Autodesk Inventor part; units mm, degrees
ref_plane "YZ Plane" through (0, 0, 0) normal (1, 0, 0) x (0, 1, 0)
ref_plane "XZ Plane" through (0, 0, 0) normal (0, 1, 0) x (-1, 0, 0)
ref_plane "XY Plane" through (0, 0, 0) normal (0, 0, 1) x (1, 0, 0)
sketch "Sketch1" plane through (0, 0, 0) normal (0, 0, 1) x (1, 0, 0)
  line L0 (-160, -10) -> (160, -10)
  line L1 (160, -10) -> (160, 10) construction
  line L2 (160, 10) -> (-160, 10)
  line L3 (-160, 10) -> (-160, -10) construction
  line L4 (-160, -10) -> (160, 10) construction
  line L5 (160, -10) -> (-160, 10) construction
  arc A0 (-160, 10) -> (-160, -10) centre (-160, 0) ccw
  arc A1 (160, -10) -> (160, 10) centre (160, 0) ccw
  point P0 (0, 0)
  dimension "d0" = 320
  dimension "d1" = 20
extrude "Extrusion1" add sketch "Sketch1" along normal blind 20
sketch "Sketch3" plane through (0, 0, 20) normal (0, 0, 1) x (1, 0, 0)
  arc A0 (-160, 10) -> (-160, -10) centre (-160, 0) ccw
  circle A1 centre (-160, 0) radius 7
  point P0 (0, 0)
  dimension "d7" = 14
extrude "Extrusion3" cut sketch "Sketch3" against normal blind 15
properties part number "u_kleine_Hoehenverstellung"
The model under review builds one solid part; all positions refer to its coordinate system, in mm. A direction names the side the tool comes from. Round coordinates to 2 decimals unless told otherwise and drop trailing zeros. Order: outer loops, then holes, each group sorted by start corner. A loop starts at its lowest first (then second) coordinate and runs counter-clockwise, first axis right, second up. Notation, with made-up numbers: (48.5, -5) -> (104.5, -5) arc R20 cw to (104.5, 20) -> close; hole circle Ø11 at (44, 89). An arc over 180 degrees is marked (long way). Use a Markdown table: item, result.
Q1. Tool access review of faces 4 (the flat face through (-160, 0, 5)), 5 (the flat face through (-2, 0, 0)): name each direction out of +Z, -Z, +X, -X, +Y, -Y from which nothing blocks a thin tool from reaching the whole face with its end or side.
Values:
| item | result |
|---|---|
| face 4 | +Z |
| face 5 | -Z, +X, -X, +Y, -Y |
Q2. For line 1 (Y direction, x = -160, z = 16); line 2 (X direction, y = 0, z = 3.5); line 3 (X direction, y = 5.25, z = 15), list the stretches that pass through material, from the lowest coordinate up.
Values:
| item | result |
|---|---|
| line 1 | y = -10 to -7, 7 to 10 |
| line 2 | x = -170 to 170 |
| line 3 | x = -168.51 to -164.63, -155.37 to 168.51 |
Q3. We need section A-A on y = 0. Write out the cut boundary in (x, z).
Values:
| item | result |
|---|---|
| outline | (-170, 0) -> (170, 0) -> (170, 20) -> (-153, 20) -> (-153, 5) -> (-167, 5) -> (-167, 20) -> (-170, 20) -> close |
Q4. We need section B-B on z = 15.75. Write out the cut boundary in (x, y).
Values:
| item | result |
|---|---|
| outline | (-160, -10) -> (160, -10) arc R10 ccw to (160, 10) -> (-160, 10) arc R10 ccw to start; hole circle Ø14 at (-160, 0) |
Q5. Clearance check with a flat-ended pin moving along its axis: P1, Ø1.5, axis at y = 2, z = 12.5, coming from the +X side. State where the tip first meets the part, or that it passes through.
Values:
| item | result |
|---|---|
| P1 | stops at x = 169.92 |
Q6. Mouldability with a two-part tool opening along Y and no side actions: class faces 1 (the cylindrical face through (-153.534, -2.681, 12.605)), 2 (the flat face through (-2, 0, 20)), 3 (the cylindrical face through (170, 0, 10)) as +Y half, -Y half, draft (parallel to the pull), parting line (faces both ways), or undercut.
Values:
| item | result |
|---|---|
| face 1 | undercut |
| face 2 | draft |
| face 3 | parting line |
